For this review, take the finished solid that the model builds, in its own axes (mm). Round coordinates to 2 decimals unless told otherwise and drop trailing zeros. Loops run counter-clockwise (first coordinate to the right, second up) from the corner with the lowest first, then second, coordinate; pieces in that order, holes last.
1) Wall thickness on L1, parallel to Y at x = -30.5, z = 1.85; L2, parallel to Y at x = -62, z = 2.3; L3, parallel to Y at x = -71.5, z = 2.5: over which ranges is each line inside the solid? List them lowest first.
2) Insertion check: pin 1 (1 mm diameter, centred on y = -16.5, z = 1.5, fed in from +X). The pin has a flat end and moves straight along its axis. Give the tip position at first contact, or say it passes through.
3) Mouldability with a two-part tool opening along X and no side actions: class faces 1 (the flat face through (-15.3, 107.22, 1.57)), 2 (the cylindrical face through (-83.38, 89.26, 1.57)), 3 (the flat face through (-71, 20, 3.175)), 4 (the flat face through (-123.974, 107.383, 1.565)) as pulls with the +X half, pulls with the -X half, needs draft (parallel to the pull), parting line crosses it, or undercut.
4) Take a section at C-C (x = -75). State the section outline as (y, z) points (3 decimals).
5) Take a section at D-D (y = -2). State the section outline as (x, z) points (3 decimals), then the cut area to 3 significant figures.
6) Take a section at B-B (x = -17.5). State the section outline as (y, z) points (3 decimals).
7) Take a section at A-A (y = -54.5). State the section outline as (x, z) points (3 decimals).
```python
from build123d import *

# Parameters (mm, degrees)
F0_R     = 1.7859375
F0_R_2   = 10.795
F1_DEPTH = 3.175
F2_R     = 2.54


with BuildPart() as f1:
    # F0 (on Top) → F1 (new body)
    with BuildSketch(Plane.XY):
        Polygon((-136.4652514458, -19.908263123), (-136.4652514458, -77.058263123), (-3.1152514458, -77.058263123), (-3.1152514458, -19.908263123), (-34.8652514458, -19.908263123), (-34.8652514458, -13.558263123), (-53.9152514458, -13.558263123), (-53.9152514458, 30.891736877), (-34.8652514458, 30.891736877), (-34.8652514458, 37.241736877), (-3.1152514458, 37.241736877), (-3.1152514458, 100.741736877), (-27.0015158653, 113.441736877), (-112.5789870262, 113.441736877), (-136.4652514458, 100.741736877), (-136.4652514458, 37.241736877), (-104.7152514458, 37.241736877), (-104.7152514458, 30.891736877), (-85.6652514458, 30.891736877), (-85.6652514458, -13.558263123), (-104.7152514458, -13.558263123), (-104.7152514458, -19.908263123), align=None)
        with Locations((-85.0302514458, -61.818263123)):
            Circle(F0_R, mode=Mode.SUBTRACT)
        with Locations((-57.5474514458, -74.569063123)):
            Circle(F0_R, mode=Mode.SUBTRACT)
        with Locations((-69.7902514458, -61.818263123)):
            Circle(F0_R_2, mode=Mode.SUBTRACT)
        with Locations((-54.5502514458, -61.818263123)):
            Circle(F0_R, mode=Mode.SUBTRACT)
        with Locations((-5.6552514458, -69.870063123)):
            Circle(F0_R, mode=Mode.SUBTRACT)
        with Locations((-5.6552514458, -41.980863123)):
            Circle(F0_R, mode=Mode.SUBTRACT)
        with Locations((-97.5715014458, 108.361736877)):
            Circle(F0_R, mode=Mode.SUBTRACT)
        with Locations((-85.0302514458, 89.946736877)):
            Circle(F0_R, mode=Mode.SUBTRACT)
        with Locations((-69.7902514458, 89.946736877)):
            Circle(F0_R_2, mode=Mode.SUBTRACT)
        with Locations((-54.5502514458, 89.946736877)):
            Circle(F0_R, mode=Mode.SUBTRACT)
        with Locations((-42.0090014458, 108.361736877)):
            Circle(F0_R, mode=Mode.SUBTRACT)
    extrude(amount=F1_DEPTH)

    # F2
    f2_edges = [f1.edges().sort_by_distance(p)[0] for p in [
        (-34.865251, 37.241737, 1.5875),
        (-3.115251, -19.908263, 1.5875),
        (-3.115251, 37.241737, 1.5875),
        (-3.115251, -77.058263, 1.5875),
        (-136.465251, -77.058263, 1.5875),
        (-3.115251, 100.741737, 1.5875),
        (-27.001516, 113.441737, 1.5875),
        (-112.578987, 113.441737, 1.5875),
        (-136.465251, 100.741737, 1.5875),
        (-136.465251, 37.241737, 1.5875),
        (-104.715251, 37.241737, 1.5875),
        (-136.465251, -19.908263, 1.5875),
        (-53.915251, 30.891737, 1.5875),
        (-53.915251, -13.558263, 1.5875),
        (-85.665251, -13.558263, 1.5875),
        (-104.715251, -13.558263, 1.5875),
        (-85.665251, 30.891737, 1.5875),
        (-34.865251, -13.558263, 1.5875),
        (-104.715251, 30.891737, 1.5875),
        (-104.715251, -19.908263, 1.5875),
        (-34.865251, -19.908263, 1.5875),
        (-34.865251, 30.891737, 1.5875),
    ]]
    fillet(f2_edges, radius=F2_R)


solid = f1.part
```
Response:
1. L1: y = -77.06 to -19.91, 37.24 to 113.44
1. L2: y = -77.06 to -69.29, -54.35 to 82.47, 97.42 to 113.44
1. L3: y = -77.06 to -72.48, -51.16 to 79.29, 100.61 to 113.44
2. pin 1: stops at x = -34.87
3. face 1: pulls with the +X half
3. face 2: undercut
3. face 3: needs draft
3. face 4: pulls with the -X half
4. outline: (-77.058, 0) - (-71.273, 0) - (-71.273, 3.175) - (-77.058, 3.175) - close; (-52.364, 0) - (80.492, 0) - (80.492, 3.175) - (-52.364, 3.175) - close; (99.401, 0) - (113.442, 0) - (113.442, 3.175) - (99.401, 3.175) - close
5. outline: (-85.665, 0) - (-53.915, 0) - (-53.915, 3.175) - (-85.665, 3.175) - close
5. area: 101 mm2
6. outline: (-77.058, 0) - (-19.908, 0) - (-19.908, 3.175) - (-77.058, 3.175) - close; (37.242, 0) - (108.39, 0) - (108.39, 3.175) - (37.242, 3.175) - close
7. outline: (-136.465, 0) - (-77.726, 0) - (-77.726, 3.175) - (-136.465, 3.175) - close; (-61.855, 0) - (-3.115, 0) - (-3.115, 3.175) - (-61.855, 3.175) - close
